Design review of the part built by this model. Coordinates are the model's own, in mm. Face numbers are marked on the shaded views. A direction names the side the tool comes from. Round coordinates to 2 decimals unless told otherwise and drop trailing zeros. Loops run counter-clockwise (first coordinate to the right, second up) from the corner with the lowest first, then second, coordinate; pieces in that order, holes last. Notation, with made-up numbers: (-20, -39.75) - (32, -39.75) arc R25 cw to (32, -12.75) - close; hole circle Ø11 at (2, 59). An arc over 180 degrees is marked (long way). Use one line per item in the form item = value. Start each with the question number.
(1) We need section B-B, the plane x = -10. Give the number of separate pieces and of enclosed holes in the cut face, then the cut area to 3 significant figures.
(2) We need section C-C, the plane z = -8. Write out the cut boundary in (x, y), then the cut area to 3 significant figures.
(3) We need section D-D, the plane y = 13.75. Write out the cut boundary in (x, z), then the cut area to 3 significant figures.
(4) For pin 1 (4 mm diameter, centred on y = 13, z = -9, fed in from -X); pin 2 (0.8 mm diameter, centred on x = 0, y = 7, fed in from -Z); pin 3 (2 mm diameter, centred on x = 1.5, y = 10, fed in from -Z), all flat-tipped, find the tip position at first contact; note any pin that passes through.
(5) We need section A-A, the plane y = 2.75. Write out the cut boundary in (x, z), then the cut area to 3 significant figures.
(6) The part is to be moulded in two halves that separate along X. For the marked faces 1, 2, 3 and 4, say which applies: released by +X, released by -X, zero draft, split by the parting line, or undercut.
(7) Wall thickness on probe 1 along X at (y, z) = (10.5, 0.5); probe 2 along X at (y, z) = (8.75, 20); probe 3 along Z at (x, y) = (8, 3.75): over which ranges is each line inside the solid? List them lowest first. Write a range as [from, to].
(8) Machinability: for the marked faces 5, 6, 7 and 8, which of the approach directions +Z, -Z, +X, -X, +Y, -Y give a long, thin tool a straight path to every point of the face, cutting with its end or side? Answer none if there is none.
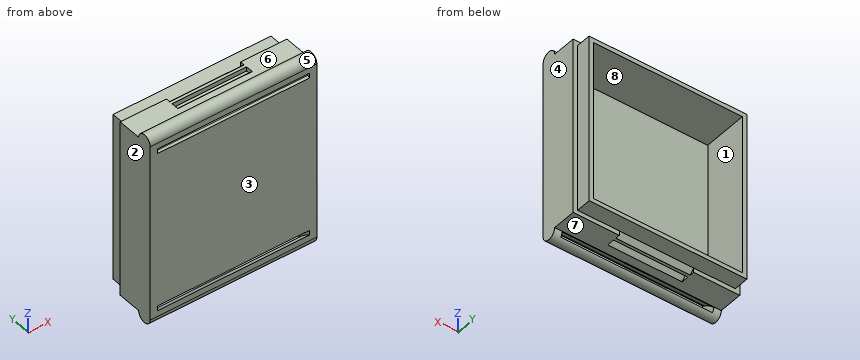
from build123d import *

# Parameters (mm, degrees)
SKETCH1_W                       = 56
SKETCH1_H                       = 60
SKETCH1_W_2                     = 50
SKETCH1_H_2                     = 54
BOSS_EXTRUDE1_DEPTH             = 10
SKETCH2_W                       = 56
SKETCH2_H                       = 60
BOSS_EXTRUDE2_DEPTH             = 3
CUT_EXTRUDE1_DEPTH              = 12.5
BOSS_EXTRUDE4_REACH             = 44.237
BOSS_EXTRUDE4_DIRECTION_2_REACH = 44.237
BOSS_EXTRUDE5_DEPTH             = 25.5
SKETCH7_W                       = 53
SKETCH7_H                       = 57
SKETCH7_W_2                     = 50
SKETCH7_H_2                     = 54
BOSS_EXTRUDE6_DEPTH             = 5


with BuildPart() as part:
    # Sketch1 → Boss-Extrude1 (new body)
    with BuildSketch(Plane(origin=(0, 0, 0), x_dir=(1, 0, 0), z_dir=(0, 1, 0))):
        Rectangle(SKETCH1_W, SKETCH1_H)
        Rectangle(SKETCH1_W_2, SKETCH1_H_2, mode=Mode.SUBTRACT)
    extrude(amount=BOSS_EXTRUDE1_DEPTH)

    # Sketch2 → Boss-Extrude2 (add)
    with BuildSketch(Plane.XZ):
        Rectangle(SKETCH2_W, SKETCH2_H)
    extrude(amount=BOSS_EXTRUDE2_DEPTH)

    # Sketch3 → Cut-Extrude1 (cut, symmetric)
    with BuildSketch(Plane(origin=(0, 0, 0), x_dir=(0, 0, -1), z_dir=(1, 0, 0))):
        Polygon((-28.5, 10), (-31, 10), (-31, 4), (-28.5, 6.5), (-28.5, 7.5), (-30, 7.5), (-30, 8.5), align=None)
    cut_extrude1 = extrude(amount=CUT_EXTRUDE1_DEPTH, both=True, mode=Mode.SUBTRACT)

    # Mirror1: Cut-Extrude1 across plane
    add(cut_extrude1.mirror(Plane.XY), mode=Mode.SUBTRACT)

    # Boss-Extrude4: up to this face of the body (flat: up to its plane)
    boss_extrude4_end = Plane(part.part.faces().sort_by_distance((28, 3.5, 0))[0])
    # Sketch4 → Boss-Extrude4 (add, up to the picked face)
    with BuildSketch(Plane(origin=(0, 0, 0), x_dir=(0, 0, -1), z_dir=(1, 0, 0)), mode=Mode.PRIVATE) as boss_extrude4_sk1:
        with BuildLine():
            Line((30, 2), (30, -3))
            ThreePointArc((30, -3), (32.5, -0.5), (30, 2))
        make_face()
    boss_extrude4_tool1 = split(extrude(boss_extrude4_sk1.sketch, amount=BOSS_EXTRUDE4_REACH, mode=Mode.PRIVATE), bisect_by=boss_extrude4_end, keep=Keep.BOTH, mode=Mode.PRIVATE)
    boss_extrude4 = boss_extrude4_tool1.solids().sort_by(Axis((0, -0.5, -31.061033), (1, 0, 0)))[0]
    add(boss_extrude4)

    # Boss-Extrude4 direction 2: up to this face of the body (flat: up to its plane)
    boss_extrude4_direction_2_end = Plane(part.part.faces().sort_by_distance((-28, 3.5, 0))[0])
    # Sketch4 → Boss-Extrude4 direction 2 (add, up to the picked face)
    with BuildSketch(Plane(origin=(0, 0, 0), x_dir=(0, 0, -1), z_dir=(1, 0, 0)), mode=Mode.PRIVATE) as boss_extrude4_direction_2_sk1:
        with BuildLine():
            Line((30, 2), (30, -3))
            ThreePointArc((30, -3), (32.5, -0.5), (30, 2))
        make_face()
    boss_extrude4_direction_2_tool1 = split(extrude(boss_extrude4_direction_2_sk1.sketch, amount=-BOSS_EXTRUDE4_DIRECTION_2_REACH, mode=Mode.PRIVATE), bisect_by=boss_extrude4_direction_2_end, keep=Keep.BOTH, mode=Mode.PRIVATE)
    boss_extrude4_direction_2 = boss_extrude4_direction_2_tool1.solids().sort_by(Axis((0, -0.5, -31.061033), (-1, 0, 0)))[0]
    add(boss_extrude4_direction_2)

    # Mirror3: Boss-Extrude4, Boss-Extrude4 direction 2 across plane
    add(boss_extrude4.mirror(Plane.XY))
    add(boss_extrude4_direction_2.mirror(Plane.XY))

    # Sketch7 → Boss-Extrude6 (add)
    with BuildSketch(Plane(origin=(0, 10, 0), x_dir=(1, 0, 0), z_dir=(0, 1, 0))):
        Rectangle(SKETCH7_W, SKETCH7_H)
        Rectangle(SKETCH7_W_2, SKETCH7_H_2, mode=Mode.SUBTRACT)
    extrude(amount=BOSS_EXTRUDE6_DEPTH)


with BuildPart() as body_2:
    # Sketch5 → Boss-Extrude5 (new, symmetric)
    with BuildSketch(Plane(origin=(0, 0, 0), x_dir=(0, 0, -1), z_dir=(1, 0, 0))):
        with BuildLine():
            Line((26.787564435, -2.3), (26.383419246, -3))
            Line((26.383419246, -3), (28, -3))
            ThreePointArc((28, -3), (29.996934481, -0.214678652), (32.5, 2.126352177))
            Line((32.5, 2.126352177), (32.5, 3.852866185))
            ThreePointArc((32.5, 3.852866185), (29.29668765, 1.098682153), (26.787564435, -2.3))
        make_face()
    extrude(amount=BOSS_EXTRUDE5_DEPTH, both=True)


with BuildPart() as body_3:
    # Mirror2: mirrored copy
    add(body_2.part.mirror(Plane.XY))


with BuildPart() as part_1:
    add(part.part)

    # Combine1: cut body 2, body 3
    add(body_2.part, mode=Mode.SUBTRACT)
    add(body_3.part, mode=Mode.SUBTRACT)


solid = part_1.part
Data:
q1.separate_pieces = 3
q1.enclosed_holes = 0
q1.area = 250 mm^2
q2.outline = (-28, -3) - (28, -3) - (28, 10) - (26.5, 10) - (26.5, 15) - (25, 15) - (25, 0) - (-25, 0) - (-25, 15) - (-26.5, 15) - (-26.5, 10) - (-28, 10) - close
q2.area = 243 mm^2
q3.outline = (-26.5, -28.5) - (26.5, -28.5) - (26.5, 28.5) - (-26.5, 28.5) - close; hole (-25, -27) - (25, -27) - (25, 27) - (-25, 27) - close
q3.area = 321 mm^2
q4.pin_1 = -26.5
q4.pin_2 = -28.5
q4.pin_3 = -29.5
q5.outline = (-28, -30) - (28, -30) - (28, 30) - (-28, 30) - close; hole (-25, -27) - (25, -27) - (25, 27) - (-25, 27) - close
q5.area = 660 mm^2
q6.face_1 = undercut
q6.face_2 = released by -X
q6.face_3 = zero draft
q6.face_4 = released by +X
q7.probe_1 = [-26.5, -25], [25, 26.5]
q7.probe_2 = [-28, -25], [25, 28]
q7.probe_3 = [-30, -27], [27, 30]
q8.face_5 = +Z, +X, -X
q8.face_6 = +Z, +X, -X, +Y
q8.face_7 = -Z, +X, -X, +Y
q8.face_8 = +Y
